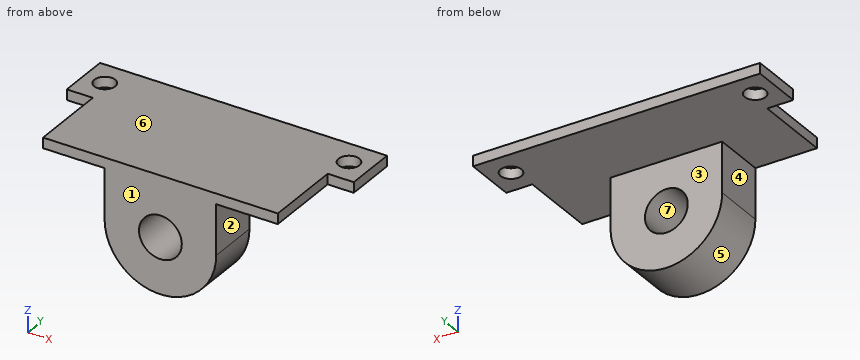
```python
from build123d import *

# Parameters (mm, degrees)
BOSS_EXTRUDE1_START = 4
SKETCH1_W           = 45
SKETCH1_H           = 15
SKETCH1_W_2         = 55
SKETCH1_H_2         = 10
SKETCH1_R           = 2
BOSS_EXTRUDE1_DEPTH = 2
SKETCH2_R           = 10.7
SKETCH2_R_2         = 4.1
BOSS_EXTRUDE2_DEPTH = 10
BOSS_EXTRUDE3_START = -10
BOSS_EXTRUDE3_DEPTH = 10


with BuildPart() as part:
    # Sketch1 → Boss-Extrude1 (new body)
    # profile 1 of 2: a face of its own
    with BuildSketch(Plane.XY.offset(BOSS_EXTRUDE1_START)):
        with Locations((15.006572053, -17.5)):
            Rectangle(SKETCH1_W, SKETCH1_H)
    # profile 2 of 2: a face of its own
    with BuildSketch(Plane.XY.offset(BOSS_EXTRUDE1_START)):
        with Locations((15.006572053, -5)):
            Rectangle(SKETCH1_W_2, SKETCH1_H_2)
        with Locations(Location((-8.393427947, -5, 0), (0, 0, 90))):
            Circle(SKETCH1_R, mode=Mode.SUBTRACT)
        with Locations(Location((38.406572053, -5, 0), (0, 0, 90))):
            Circle(SKETCH1_R, mode=Mode.SUBTRACT)
    extrude(amount=BOSS_EXTRUDE1_DEPTH)

    # Sketch2 → Boss-Extrude2 (add)
    with BuildSketch(Plane(origin=(0, -25, 0), x_dir=(1, 0, 0), z_dir=(0, 1, 0))):
        with Locations((15.006572053, 5.6)):
            Circle(SKETCH2_R)
        with Locations(Location((15.006572053, 5.6, 0), (0, 0, 270))):
            Circle(SKETCH2_R_2, mode=Mode.SUBTRACT)
    extrude(amount=BOSS_EXTRUDE2_DEPTH)

    # Sketch3 → Boss-Extrude3 (add)
    with BuildSketch(Plane(origin=(0, -15, 0), x_dir=(1, 0, 0), z_dir=(0, 1, 0)).offset(BOSS_EXTRUDE3_START)):
        with BuildLine():
            Line((25.706572053, 5.6), (19.106572053, 5.6))
            ThreePointArc((19.106572053, 5.6), (15.006572053, 1.5), (10.906572053, 5.6))
            Line((10.906572053, 5.6), (4.306572053, 5.6))
            ThreePointArc((4.306572053, 5.6), (5.922177371, -0.053651322), (10.281109113, -4))
            Line((10.281109113, -4), (19.732034993, -4))
            ThreePointArc((19.732034993, -4), (24.090966734, -0.053651322), (25.706572053, 5.6))
        make_face()
        with BuildLine():
            Line((25.706572053, -6), (25.706572053, 5.6))
            ThreePointArc((25.706572053, 5.6), (24.090966734, -0.053651322), (19.732034993, -4))
            Line((19.732034993, -4), (10.281109113, -4))
            ThreePointArc((10.281109113, -4), (5.922177371, -0.053651322), (4.306572053, 5.6))
            Line((4.306572053, 5.6), (4.306572053, -6))
            Line((4.306572053, -6), (25.706572053, -6))
        make_face()
    extrude(amount=BOSS_EXTRUDE3_DEPTH)


solid = part.part
```
Check sheet for the modelled part. Datum: model origin and axes. Units: mm. Face numbers are marked on the shaded views. A direction names the side the tool comes from. Round coordinates to 2 decimals unless told otherwise and drop trailing zeros. Order: outer loops, then holes, each group sorted by start corner. A loop starts at its lowest first (then second) coordinate and runs counter-clockwise, first axis right, second up. Notation, with made-up numbers: (-23, 56) - (14, 56) arc R22 ccw to (14, 69) - close; hole circle Ø9 at (57.5, 50.5). An arc over 180 degrees is marked (long way). Answer as CSV lines item,"result". Start each with the question number.
1) Section check B-B (y = -18). Record the cut outline in (x, z), then the cut area to 3 significant figures.
2) Scan lines: probe 1 along X at (y, z) = (-5, 5.5); probe 2 along Z at (x, y) = (-0.5, -13.75); probe 3 along X at (y, z) = (-18.5, 0.75). Record each from-to range of solid material in increasing order.
3) Tool access check on the marked faces 1, 2 and 3. Record the directions out of +Z, -Z, +X, -X, +Y, -Y that give a thin tool (end or side, any length) a straight path to the whole face; none if there is none.
4) Depth check by flat-ended pin: pin 1 (7.5 mm diameter, centred on y = -20.5, z = -1, fed in from +X); pin 2 (13 mm diameter, centred on x = 15.01, z = -5.6, fed in from -Y); pin 3 (2 mm diameter, centred on y = -16, z = 5.5, fed in from +X); pin 4 (2 mm diameter, centred on y = -17.5, z = 0, fed in from -X). Enter the tip coordinate at first touch or a pass-through.
5) Section check C-C (x = 2). Record the cut outline in (y, z).
6) Section check A-A (y = -5). Record the cut outline in (x, z).
7) Draft check along Z on the marked faces 4, 5, 6 and 7. Enter one of: +Z half, -Z half, draft (parallel to the pull), parting line (faces both ways), or undercut.
8) Section check D-D (z = -11). Record the cut outline in (x, y).
Determined:
1,outline,"(-7.49, 4) - (4.31, 4) - (4.31, -5.6) arc R10.7 ccw to (25.71, -5.6) - (25.71, 4) - (37.51, 4) - (37.51, 6) - (-7.49, 6) - close; hole circle Ø8.2 at (15.01, -5.6)"
1,area,"422 mm^2"
2,probe 1,"-12.49 to -10.39, -6.39 to 36.41, 40.41 to 42.51"
2,probe 2,"4 to 6"
2,probe 3,"4.31 to 25.71"
3,face 1,"+Z, -Z, +X, -X, -Y"
3,face 2,"-Z, +X, +Y, -Y"
3,face 3,"-Z, +X, -X, +Y"
4,pin 1,"x = 25.71"
4,pin 2,"y = -25"
4,pin 3,"x = 37.51"
4,pin 4,"x = 4.31"
5,outline,"(-25, 4) - (0, 4) - (0, 6) - (-25, 6) - close"
6,outline,"(-12.49, 4) - (-10.39, 4) - (-10.39, 6) - (-12.49, 6) - close; (-6.39, 4) - (36.41, 4) - (36.41, 6) - (-6.39, 6) - close; (40.41, 4) - (42.51, 4) - (42.51, 6) - (40.41, 6) - close"
7,face 4,"draft"
7,face 5,"-Z half"
7,face 6,"+Z half"
7,face 7,"undercut"
8,outline,"(5.77, -25) - (24.24, -25) - (24.24, -15) - (5.77, -15) - close"
